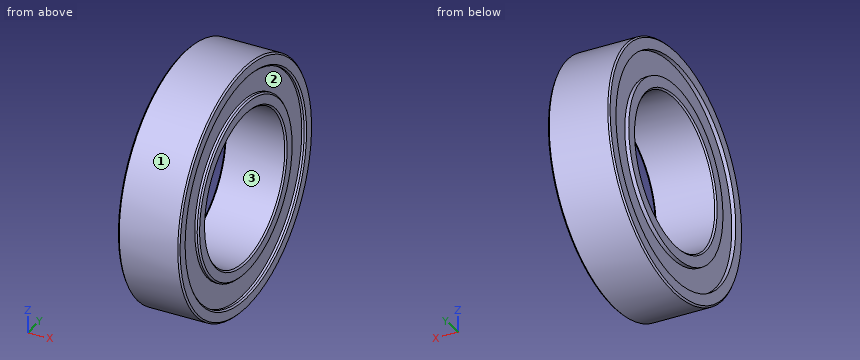
from build123d import *

# Parameters (mm, degrees)
SKETCH1_R             = 5.61975
SKETCH1_R_2           = 4.826
BOSS_EXTRUDE1_DEPTH   = 1.984375
SKETCH1_R_3           = 7.9375
SKETCH1_R_4           = 7.14375
BOSS_EXTRUDE1_2_DEPTH = 1.984375
SKETCH2_R             = 7.14375
SKETCH2_R_2           = 5.61975
BOSS_EXTRUDE2_DEPTH   = 1.730375
CHAMFER1_SIZE         = 0.09921875


with BuildPart() as part:
    # Sketch1 → Boss-Extrude1 (new, symmetric)
    with BuildSketch(Plane(origin=(0, 0, 0), x_dir=(0, 0, -1), z_dir=(1, 0, 0))):
        Circle(SKETCH1_R)
        Circle(SKETCH1_R_2, mode=Mode.SUBTRACT)
    extrude(amount=BOSS_EXTRUDE1_DEPTH, both=True)



with BuildPart() as body_2:
    # Sketch1 → Boss-Extrude1 2 (new, symmetric)
    with BuildSketch(Plane(origin=(0, 0, 0), x_dir=(0, 0, -1), z_dir=(1, 0, 0))):
        Circle(SKETCH1_R_3)
        Circle(SKETCH1_R_4, mode=Mode.SUBTRACT)
    extrude(amount=BOSS_EXTRUDE1_2_DEPTH, both=True)


with BuildPart() as part_1:
    add(part.part)

    add(body_2.part)  # Boss-Extrude2 merges body 2
    # Sketch2 → Boss-Extrude2 (add, symmetric)
    with BuildSketch(Plane(origin=(0, 0, 0), x_dir=(0, 0, -1), z_dir=(1, 0, 0))):
        Circle(SKETCH2_R)
        Circle(SKETCH2_R_2, mode=Mode.SUBTRACT)
    extrude(amount=BOSS_EXTRUDE2_DEPTH, both=True)

    # Chamfer1
    chamfer1_edges = [part_1.edges().sort_by_distance(p)[0] for p in [
        (1.984375, 0, 5.61975),
        (1.984375, 0, 7.14375),
        (-1.984375, 0, 7.9375),
        (1.984375, 0, 7.9375),
        (-1.984375, 0, 4.826),
        (1.984375, 0, 4.826),
    ]]
    chamfer(chamfer1_edges, length=CHAMFER1_SIZE)


solid = part_1.part
Could you check a few things on this model? Use its own coordinates, in mm. Face numbers are marked on the shaded views. Give positions to 0.01 mm unless a question says otherwise; leave off trailing zeros. Order: outer loops, then holes, each group sorted by start corner. A loop starts at its lowest first (then second) coordinate and runs counter-clockwise, first axis right, second up.
1. Thinking about a two-plate mould opening in Y: for the marked faces 1, 2 and 3, which applies, +Y half, -Y half, draft (parallel to the pull), parting line (faces both ways), or undercut?
Answers below:
face 1: parting line
face 2: undercut
face 3: undercut
2. Suppose I cut it at A-A (x = 0.9). Write out the boundary of the cut face in (y, z) (1 decimal).
Answers below:
outline: circle Ø15.9 at (0, 0); hole circle Ø9.7 at (0, 0)
3. For pin 1 (2 mm diameter, centred on y = -2.5, z = 1.5, fed in from +X); pin 2 (1 mm diameter, centred on x = 1, z = -3, fed in from -Y), each with a flat end and sliding along its axis, tell me the tip position at first contact or that it passes through.
Answers below:
pin 1: passes through
pin 2: stops at y = -7.53
4. I need wall thicknesses on L1, parallel to Y at x = 1.8, z = 0; L2, parallel to Y at x = -0.15, z = 0; L3, parallel to Y at x = 1.8, z = -3.5. Which ranges of each line are inside material? Lowest first, please.
Answers below:
L1: y = -7.94 to -7.14, -5.62 to -4.83, 4.83 to 5.62, 7.14 to 7.94
L2: y = -7.94 to -4.83, 4.83 to 7.94
L3: y = -7.12 to -6.23, -4.4 to -3.32, 3.32 to 4.4, 6.23 to 7.12
